from build123d import *

# Parameters (mm, degrees)
SKETCH1_W           = 3.175
SKETCH1_H           = 395.409928
BOSS_EXTRUDE1_DEPTH = 228.6
CUT_EXTRUDE1_DEPTH  = 457.746156838
BOSS_EXTRUDE4_REACH = 458.746
BOSS_EXTRUDE5_DEPTH = 50.165
BOSS_EXTRUDE8_REACH = 449.107


with BuildPart() as part:
    # Sketch1 → Boss-Extrude1 (new body)
    with BuildSketch(Plane(origin=(0, 0, 0), x_dir=(1, 0, 0), z_dir=(0, 1, 0))):
        with Locations((1.5875, 197.704964)):
            Rectangle(SKETCH1_W, SKETCH1_H)
    extrude(amount=BOSS_EXTRUDE1_DEPTH)

    # Sketch2 → Cut-Extrude1 (cut, through all)
    with BuildSketch(Plane(origin=(3.175, 0, 0), x_dir=(0, 0, -1), z_dir=(1, 0, 0))):
        Polygon((0, 0), (395.409928, 71.795894), (395.409928, 0), align=None)
    extrude(amount=-CUT_EXTRUDE1_DEPTH, mode=Mode.SUBTRACT)

    # Boss-Extrude4: up to this plane
    boss_extrude4_end = Plane(origin=(0, 0, 0), z_dir=(0, 0.9839122845611679, 0.17865222161961358))
    # Sketch8 → Boss-Extrude4 (add, up to the surface)
    with BuildSketch(Plane(origin=(0, 228.6, 0), x_dir=(1, 0, 0), z_dir=(0, 1, 0)), mode=Mode.PRIVATE) as boss_extrude4_sk1:
        Polygon((0, 395.409928), (34.459069357, 408.410752554), (35.579830094, 405.440143126), (0, 392.016474486), align=None)
    boss_extrude4_tool1 = split(extrude(boss_extrude4_sk1.sketch, amount=-BOSS_EXTRUDE4_REACH, mode=Mode.PRIVATE), bisect_by=boss_extrude4_end, keep=Keep.BOTH, mode=Mode.PRIVATE)
    add(boss_extrude4_tool1.solids().sort_by_distance((17.511219, 228.6, -400.310838))[0])

    # Sketch9 → Boss-Extrude5 (add)
    with BuildSketch(Plane(origin=(0, 228.6, 0), x_dir=(1, 0, 0), z_dir=(0, 1, 0))):
        Polygon((3.175, 0), (-26.531094273, -11.207607374), (-27.65185501, -8.236997947), (3.175, 3.393453514), align=None)
    extrude(amount=-BOSS_EXTRUDE5_DEPTH)

    # Boss-Extrude8: up to this plane
    boss_extrude8_end = Plane(origin=(0, 0, 0), z_dir=(0, 0.9839122845611679, 0.17865222161961358))
    # Sketch13 → Boss-Extrude8 (add, up to the surface)
    with BuildSketch(Plane.XZ.offset(-178.435), mode=Mode.PRIVATE) as boss_extrude8_sk1:
        Polygon((0, 0), (10.19197679, 27.014135421), (13.162586217, 25.893374684), (1.954978843, -3.812719589), align=None)
    boss_extrude8_tool1 = split(extrude(boss_extrude8_sk1.sketch, amount=BOSS_EXTRUDE8_REACH, mode=Mode.PRIVATE), bisect_by=boss_extrude8_end, keep=Keep.BOTH, mode=Mode.PRIVATE)
    add(boss_extrude8_tool1.solids().sort_by_distance((6.346866, 178.435, 12.254186))[0])


solid = part.part
The model under review builds one solid part; all positions refer to its coordinate system, in mm. A direction names the side the tool comes from. Round coordinates to 2 decimals unless told otherwise and drop trailing zeros. Loops run counter-clockwise (first coordinate to the right, second up) from the corner with the lowest first, then second, coordinate; pieces in that order, holes last. Notation, with made-up numbers: M 62.5,-30 L 103.5,-30 A17 cw 103.5,-12 Z; hole C 49,6 d2. An arc over 180 degrees is marked long. Answer as CSV lines item,"result". Start each with the question number.
Item 1: Insertion check: P1, Ø4, axis at x = 6.5, z = 9.5, coming from the +Y side (3 decimals); P2, Ø12, axis at x = 8, z = -157.5, coming from the -Y side; P3, Ø1, axis at x = 18.5, y = 98.5, coming from the -Z side. Each pin has a flat end and moves straight along its axis. Give the tip position at first contact, or say it passes through.
Item 2: Mouldability with a two-part tool opening along Z and no side actions: class faces 1 (the face through (16.99, 151.3, -401.82)), 2 (the face through (2, 228.6, -200)), 3 (the face through (8.239, 88.149, 12.842)) as released by +Z, released by -Z, zero draft, split by the parting line, or undercut.
Item 3: Consider section C-C (z = -265.5). Write out the cut boundary in (x, y) (3 decimals), then the cut area to 3 significant figures.
Item 4: Consider section D-D (y = 49). Write out the cut boundary in (x, z) (3 decimals).
Item 5: Wall thickness on line 1 (X direction, y = 169.5, z = -136) (3 decimals); line 2 (Y direction, x = 2, z = -235.5); line 3 (Z direction, x = 30, y = 194): over which ranges is each line inside the solid? List them lowest first. Write a range as [from, to].
Item 6: For faces 4 (the face through (7, 178.435, 13)), 5 (the face through (-14.019, 203.869, 3.094)), 6 (the face through (19.6, 151.1, -399.41)), list the 3-axis set-ups (+Z, -Z, +X, -X, +Y, -Y) from which the entire face can be reached by the end or side of a thin tool; tool diameter is ignored.
Item 7: Consider section A-A (y = 141). Write out the cut boundary in (x, z) (3 decimals).
Item 8: Consider section B-B (x = 24.5). Write out the cut boundary in (y, z), then the cut area to 3 significant figures.
Answer:
1,P1,"stops at y = 178.435"
1,P2,"stops at y = 27.95"
1,P3,"stops at z = -402.58"
2,face 1,"released by -Z"
2,face 2,"zero draft"
2,face 3,"undercut"
3,outline,"M 0,48.208 L 3.175,48.208 L 3.175,228.6 L 0,228.6 Z"
3,area,"573 mm^2"
4,outline,"M 0,-269.863 L 3.175,-269.863 L 3.175,-0.579 L 13.163,25.893 L 10.192,27.014 L 0,0 Z"
5,line 1,"x = [0, 3.175]"
5,line 2,"y = [42.76, 228.6]"
5,line 3,"z = [-406.73, -403.33]"
6,face 4,"+Z, +X, +Y"
6,face 5,"-Z, -X, +Y, -Y"
6,face 6,"+X, +Y, -Y"
7,outline,"M 0,-395.41 L 34.459,-408.411 L 35.58,-405.44 L 3.175,-393.214 L 3.175,-0.579 L 13.163,25.893 L 10.192,27.014 L 0,0 Z"
8,outline,"M 72.86,-401.26 L 73.47,-404.65 L 228.6,-404.65 L 228.6,-401.26 Z"
8,area,"527 mm^2"
